Geometry check sheet. Reference: the model listing, model coordinates, mm. Give positions to 0.01 mm unless a question says otherwise; leave off trailing zeros. Loops run counter-clockwise (first coordinate to the right, second up) from the corner with the lowest first, then second, coordinate; pieces in that order, holes last. Notation, with made-up numbers: (25.5, 55.25) - (57.5, 55.25) arc R14 cw to (57.5, 72.25) - close; hole circle Ø5 at (-27, -6.5). An arc over 180 degrees is marked (long way). Use a Markdown table: item, result. Add a question column.
1. Cross-section at A-A on y = 37. Enter the section's corners in (x, z), and give its area (3 significant figures).
2. Cross-section at B-B on z = 8.4. Enter the section's corners in (x, y).
3. Cross-section at C-C on x = 12.5. Enter the section's corners in (y, z), and give its area (3 significant figures).
4. Cross-section at D-D on z = 12.6. Enter the section's corners in (x, y), and give its area (3 significant figures).
5. Material ranges on L1, parallel to Y at x = 10, z = 11.4; L2, parallel to X at y = 37, z = 9.1; L3, parallel to X at y = 41.75, z = 9.8, recorded low to high.
6. Depth check by flat-ended pin: P1, Ø1.5, axis at x = 3.5, z = 10.5, coming from the -Y side; P2, Ø1.5, axis at x = 18, y = 42.5, coming from the +Z side. Enter the tip coordinate at first touch or a pass-through.
7. Draft check along X on faces 1 (the flat face through (10, 45, 9)), 2 (the cylindrical face through (9.2, 43.2, 10.5)), 3 (the cylindrical face through (9.09, 43.94, 10.97)). Enter one of: pulls with the +X half, pulls with the -X half, needs draft (parallel to the pull), parting line crosses it, or undercut.
from build123d import *

# Parameters (mm, degrees)
CYLINDER017_R     = 6.25
CYLINDER017_DEPTH = 10
CYLINDER016_R     = 7
CYLINDER016_DEPTH = 5
CYLINDER015_R     = 10.25
CYLINDER015_DEPTH = 1


with BuildPart() as redtmp07:
    # Cylinder017 → Cylinder017 (new body)
    with BuildSketch(Plane(origin=(0, -3, 0), x_dir=(1, 0, 0), z_dir=(0, 0, 1))):
        Circle(CYLINDER017_R)
    extrude(amount=CYLINDER017_DEPTH)


with BuildPart() as redtmp06:
    # Cylinder016 → Cylinder016 (new body)
    with BuildSketch(Plane(origin=(0, -3, 0), x_dir=(1, 0, 0), z_dir=(0, 0, 1))):
        Circle(CYLINDER016_R)
    extrude(amount=CYLINDER016_DEPTH)


with BuildPart() as redtop:
    # Cylinder015 → Cylinder015 (new body)
    with BuildSketch(Plane.XY):
        Circle(CYLINDER015_R)
    extrude(amount=CYLINDER015_DEPTH)

    # Fusion001: union RedTmp06
    add(redtmp06.part)

    # Cut010: cut RedTmp07
    add(redtmp07.part, mode=Mode.SUBTRACT)


with BuildPart() as redtop_1:
    # Cut010 placement: moved
    add(redtop.part.moved(Location((10, 40, 8))))


solid = redtop_1.part
Values found:
| question | item | result |
|---|---|---|
| 1 | outline | (0.2, 8) - (3.75, 8) - (3.75, 13) - (3, 13) - (3, 9) - (0.2, 9) - close; (16.25, 8) - (19.8, 8) - (19.8, 9) - (17, 9) - (17, 13) - (16.25, 13) - close |
| 1 | area | 13.1 mm2 |
| 2 | outline | circle Ø20.5 at (10, 40); hole circle Ø12.5 at (10, 37) |
| 3 | outline | (30.06, 8) - (31.27, 8) - (31.27, 13) - (30.46, 13) - (30.46, 9) - (30.06, 9) - close; (42.73, 8) - (49.94, 8) - (49.94, 9) - (43.54, 9) - (43.54, 13) - (42.73, 13) - close |
| 3 | area | 14.9 mm2 |
| 4 | outline | circle Ø14 at (10, 37); hole circle Ø12.5 at (10, 37) |
| 4 | area | 31.2 mm2 |
| 5 | L1 | y = 30 to 30.75, 43.25 to 44 |
| 5 | L2 | x = 3 to 3.75, 16.25 to 17 |
| 5 | L3 | x = 4.86 to 5.94, 14.06 to 15.14 |
| 6 | P1 | stops at y = 33.01 |
| 6 | P2 | stops at z = 9 |
| 7 | face 1 | needs draft |
| 7 | face 2 | undercut |
| 7 | face 3 | parting line crosses it |
